Can you work these out from the model? Positions are in its coordinate system, mm. Face numbers are marked on the shaded views. Give positions to 0.01 mm unless a question says otherwise; leave off trailing zeros. Loops run counter-clockwise (first coordinate to the right, second up) from the corner with the lowest first, then second, coordinate; pieces in that order, holes last. Notation, with made-up numbers: (67, -11) - (95, -11) arc R21 ccw to (95, 5) - close; hole circle Ø2 at (-13, -29). An arc over 180 degrees is marked (long way). Answer as a JSON object with one key per item and string values.
```python
from build123d import *

# Parameters (mm, degrees)
EXTRUDE_1_DEPTH     = 3
SKETCH_2_R          = 1.6
CUT_EXTRUDE_1_DEPTH = 45.821869662
EXTRUDE_2_DEPTH     = 3


with BuildPart() as part:
    # 草图1 → 凸台-拉伸1 (new body)
    with BuildSketch(Plane.XY):
        Polygon((0, 0), (20, 0), (20, -5), (40, -5), (40, -20), (0, -20), align=None)
    extrude(amount=EXTRUDE_1_DEPTH)

    # 草图2 → 切除-拉伸1 (cut, through all)
    with BuildSketch(Plane.XY.offset(3)):
        with Locations((5, -5)):
            Circle(SKETCH_2_R)
        with Locations((35, -8.75)):
            Circle(SKETCH_2_R)
        with Locations(Location((5, -15, 0), (0, 0, 180))):
            Circle(SKETCH_2_R)
        with Locations(Location((15, -5, 0), (0, 0, 180))):
            Circle(SKETCH_2_R)
        with Locations((15, -15)):
            Circle(SKETCH_2_R)
        with Locations(Location((35, -16.25, 0), (0, 0, 180))):
            Circle(SKETCH_2_R)
        with Locations((25, -16.25)):
            Circle(SKETCH_2_R)
        with Locations(Location((25, -8.75, 0), (0, 0, 180))):
            Circle(SKETCH_2_R)
    extrude(amount=-CUT_EXTRUDE_1_DEPTH, mode=Mode.SUBTRACT)

    # 草图4 → 凸台-拉伸2 (add)
    with BuildSketch(Plane.XY.offset(3)):
        Polygon((20, 0), (40, -5), (20, -5), align=None)
    extrude(amount=-EXTRUDE_2_DEPTH)


solid = part.part
```
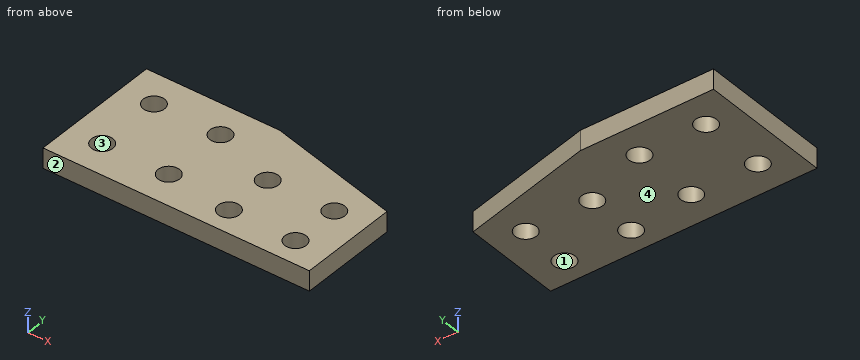
1) Imagine slicing it at D-D on x = 27. Write out the boundary of the cut face in (y, z).
Check sheet entries:
{"outline": "(-20, 0) - (-1.75, 0) - (-1.75, 3) - (-20, 3) - close"}
2) If we mould it in two halves opening along Y, with no side actions, what happens to the marked faces 1, 2, 3 and 4? For each: released by +Y, released by -Y, zero draft, split by the parting line, or undercut.
Check sheet entries:
{"face 1": "undercut", "face 2": "released by -Y", "face 3": "undercut", "face 4": "zero draft"}
3) Imagine slicing it at C-C on y = -8.75. Write out the boundary of the cut face in (x, z), and give its area (3 significant figures).
Check sheet entries:
{"outline": "(0, 0) - (23.4, 0) - (23.4, 3) - (0, 3) - close; (26.6, 0) - (33.4, 0) - (33.4, 3) - (26.6, 3) - close; (36.6, 0) - (40, 0) - (40, 3) - (36.6, 3) - close", "area": "101 mm2"}
4) Imagine slicing it at B-B on z = 1.6. Give the number of separate pieces and of enclosed holes in the cut face, and give its area (3 significant figures).
Check sheet entries:
{"separate pieces": "1", "enclosed holes": "8", "area": "686 mm2"}
5) Imagine slicing it at A-A on x = 35. Write out the boundary of the cut face in (y, z), and give its area (4 significant figures).
Check sheet entries:
{"outline": "(-20, 0) - (-17.85, 0) - (-17.85, 3) - (-20, 3) - close; (-14.65, 0) - (-10.35, 0) - (-10.35, 3) - (-14.65, 3) - close; (-7.15, 0) - (-3.75, 0) - (-3.75, 3) - (-7.15, 3) - close", "area": "29.55 mm2"}
6) I need wall thicknesses on L1, parallel to Y at x = 5, z = 2.35; L2, parallel to X at y = -14, z = 0.4; L3, parallel to X at y = -8.5, z = 2.65. Which ranges of each line are inside material? Lowest first, please.
Check sheet entries:
{"L1": "-20 to -16.6, -13.4 to -6.6, -3.4 to 0", "L2": "0 to 3.75, 6.25 to 13.75, 16.25 to 40", "L3": "0 to 23.42, 26.58 to 33.42, 36.58 to 40"}
7) I'm going to push flat-ended pins straight in: P1, Ø4, axis at x = 25, y = -16.25, coming from the -Z side; P2, Ø3, axis at x = 15, y = -15, coming from the -Z side. Where does each tip first touch, or does it pass through?
Check sheet entries:
{"P1": "z = 0", "P2": "through"}
